Geometry check sheet. Reference: the model listing, model coordinates, mm. A direction names the side the tool comes from. Give positions to 0.01 mm unless a question says otherwise; leave off trailing zeros. Write each loop counter-clockwise with the first axis right and the second up, starting at its lowest first coordinate (ties: lowest second). Pieces come first, ordered by that corner, then holes.
(1) Mould release check, pull along Y, two halves, no side actions. Record for faces 1 (the cylindrical face through (7.777, -9.686, -2.718)), 2 (the flat face through (-5, 5, -4.5)), 3 (the cylindrical face through (-4.336, -19.524, -2.218)): +Y half, -Y half, draft (parallel to the pull), parting line (faces both ways), or undercut.
(2) Cross-section at A-A (y = 0). Record the boundary of the cut face in (x, z), and give its area (3 significant figures).
(3) Cross-section at D-D (y = 14). Record the boundary of the cut face in (x, z), and give its area (3 significant figures).
(4) Cross-section at C-C (x = 17.5). Record the boundary of the cut face in (y, z).
(5) Thickness scan on line 1 along Y through (x, z) = (0, -3.95); line 2 along Y through (x, z) = (-8, -3.45); line 3 along Z through (x, y) = (2.5, -8.5). Record the ranges inside material, lowest first.
(6) Tool access check on faces 4 (the cylindrical face through (10.16, -0.09, -1.48)), 5 (the flat face through (-4.7, 9.2, 0)). Record the directions out of +Z, -Z, +X, -X, +Y, -Y that give a thin tool (end or side, any length) a straight path to the whole face; none if there is none.
(7) Depth check by flat-ended pin: P1, Ø1.5, axis at y = -3.5, z = -3, coming from the +X side; P2, Ø22.5, axis at x = -3.5, y = -2, coming from the +Z side; P3, Ø3, axis at x = -8, y = -8.07, coming from the +Z side (3 decimals); P4, Ø1, axis at y = -3.5, z = -2.5, coming from the -X side. Enter the tip coordinate at first touch or a pass-through.
(8) Cross-section at B-B (x = -5). Record the boundary of the cut face in (y, z).
Autodesk Inventor part; units mm, degrees
ref_plane "YZ Plane" through (0, 0, 0) normal (1, 0, 0) x (0, 1, 0)
ref_plane "XZ Plane" through (0, 0, 0) normal (0, 1, 0) x (-1, 0, 0)
ref_plane "XY Plane" through (0, 0, 0) normal (0, 0, 1) x (1, 0, 0)
sketch "Sketch8" plane through (0, 0, 0) normal (0, 0, 1) x (1, 0, 0)
  circle A0 centre (0, 0) radius 15
  dimension "d33" = 30
extrude "Extrusion7" add sketch "Sketch8" against normal blind 8
sketch "Sketch10" plane through (0, 0, -8) normal (0, 0, -1) x (-1, 0, 0)
  line L0 (9, 10.07) -> (-29.1, 10.07)
  arc A0 (10, 9.07) -> (9, 10.07) centre (9, 9.07) ccw
  line L1 (10, 9.07) -> (10, -9.07)
  arc A1 (9, -10.07) -> (10, -9.07) centre (9, -9.07) ccw
  line L2 (-29.1, -10.07) -> (9, -10.07)
  line L3 (-29.1, 10.07) -> (-29.1, -10.07)
  line L4 (10.4, -9.07) -> (10.4, 9.07)
  arc A2 (10.4, 9.07) -> (9, 10.47) centre (9, 9.07) ccw
  line L5 (9, 10.47) -> (-29.5, 10.47)
  line L6 (-29.5, 10.47) -> (-29.5, -10.47)
  line L7 (-29.5, -10.47) -> (9, -10.47)
  arc A3 (9, -10.47) -> (10.4, -9.07) centre (9, -9.07) ccw
  dimension "d59" = 0.4
extrude "Extrusion8" cut sketch "Sketch10" against normal blind 2 contours A0 L1 A1 L2 L3 L0 | A3 L7 L6 L5 A2 L4
sketch "Sketch11" plane through (0, 0, -6) normal (0, 0, -1) x (-1, 0, 0)
  circle A0 centre (0, 0) radius 6.4
  circle A1 centre (0, 0) radius 6.5
  point P0 (0, 0)
  dimension "d58" = 13
extrude "Extrusion9" cut sketch "Sketch11" against normal through all contours A0 | A1
sketch "Sketch13" plane through (0, 0, 0) normal (0, 0, 1) x (1, 0, 0)
  circle A0 centre (0, 0) radius 9.96
  circle A1 centre (0, 0) radius 10.16
  point P0 (0, 0)
  dimension "d44" = 0.2
extrude "Extrusion11" cut sketch "Sketch13" against normal blind 3 contours A0 | A1
sketch "Sketch14" plane through (0, 0, 0) normal (0, 0, 1) x (1, 0, 0)
  circle A0 centre (6.9, 8) radius 0.7835
  circle A1 centre (6.9, -8) radius 0.7835
  circle A2 centre (-8, 8.07) radius 1
  circle A3 centre (-8, -8.07) radius 1
  point P0 (0, 0)
hole "Hole2" at (6.9, 8, 0) at (-8, 8.07, 0) at (-8, -8.07, 0) at (6.9, -8, 0) direction (0, 0, -1) diameter 2.1 end through all
sketch "Sketch15" plane through (0, 0, 0) normal (0, 0, 1) x (1, 0, 0)
  arc A0 (7.3255, 7.0401) -> (5.888, 8.2799) centre (6.9, 8) ccw
  arc A1 (5.888, -8.2799) -> (7.3255, -7.0401) centre (6.9, -8) ccw
  circle A2 centre (-8, 8.07) radius 1.05
  circle A3 centre (-8, -8.07) radius 1.05
  circle A4 centre (6.9, 8) radius 1.9
  circle A5 centre (6.9, -8) radius 1.9
  circle A6 centre (-8, -8.07) radius 1.9
  circle A7 centre (-8, 8.07) radius 1.9
  point P0 (0, 0)
  dimension "d54" = 3.8
extrude "Extrusion12" cut sketch "Sketch15" against normal blind 4.5 contours A2 | A3 | A4 | A5 | A6 | A7
fillet "Fillet2" radius 0.5 8 edges at (5.1562, 8.7544, -1.5) (7.9023, 6.3859, -1.5) (-6.1008, 8.1244, -1.5) (-8.071, 6.1713, -1.5) (-8.071, -6.1713, -1.5) (-6.1008, -8.1244, -1.5) (5.1562, -8.7544, -1.5) (7.9023, -6.3859, -1.5)
sketch "Sketch16" plane through (0, 0, -8) normal (0, 0, -1) x (-1, 0, 0)
  circle A0 centre (-6.9, -8) radius 1.05
  circle A1 centre (8, -8.07) radius 1.05
  circle A2 centre (8, 8.07) radius 1.05
  circle A3 centre (-6.9, 8) radius 1.05
  circle A4 centre (0, 0) radius 6.5
  arc A5 (-10.7415, 10.47) -> (-10.7415, -10.47) centre (0, 0) ccw
  line L0 (9, -10.47) -> (-10.7415, -10.47)
  arc A6 (9, -10.47) -> (10.4, -9.07) centre (9, -9.07) ccw
  line L1 (10.4, 9.07) -> (10.4, -9.07)
  arc A7 (10.4, 9.07) -> (9, 10.47) centre (9, 9.07) ccw
  line L2 (-10.7415, 10.47) -> (9, 10.47)
  line L3 (-10.7415, 10.47) -> (9, 10.47)
  arc A8 (10.4, 9.07) -> (9, 10.47) centre (9, 9.07) ccw
  line L4 (10.4, 9.07) -> (10.4, -9.07)
  arc A9 (9, -10.47) -> (10.4, -9.07) centre (9, -9.07) ccw
  line L5 (9, -10.47) -> (-10.7415, -10.47)
  arc A10 (-10.7415, -10.47) -> (-10.7415, 10.47) centre (0, 0) ccw
extrude "Extrusion14" cut sketch "Sketch16" against normal blind 3.5
sketch "Sketch19" plane through (0, 0, 0) normal (0, 0, 1) x (1, 0, 0)
  circle A0 centre (0, 0) radius 15
  circle A1 centre (0, 0) radius 20
  dimension "d67" = 30
  dimension "d68" = 40
extrude "Extrusion16" add sketch "Sketch19" against normal blind 4.5
properties part number "frame_motor_support" material "Aluminum 6061-AHC"
Reply:
1. face 1: undercut
1. face 2: draft
1. face 3: parting line
2. outline: (-20, -4.5) - (-6.5, -4.5) - (-6.5, -3) - (-10.16, -3) - (-10.16, 0) - (-20, 0) - close; (6.5, -4.5) - (20, -4.5) - (20, 0) - (10.16, 0) - (10.16, -3) - (6.5, -3) - close
2. area: 99.5 mm2
3. outline: (-14.28, -4.5) - (14.28, -4.5) - (14.28, 0) - (-14.28, 0) - close
3. area: 129 mm2
4. outline: (-9.68, -4.5) - (9.68, -4.5) - (9.68, 0) - (-9.68, 0) - close
5. line 1: y = -20 to -6.5, 6.5 to 20
5. line 2: y = -18.33 to -9.97, -6.17 to 6.17, 9.97 to 18.33
5. line 3: z = -4.5 to -3
6. face 4: +Z
6. face 5: +Z, +X, -X, +Y, -Y
7. P1: stops at x = 19.81
7. P2: stops at z = 0
7. P3: passes through
7. P4: stops at x = -19.77
8. outline: (-19.36, -4.5) - (-4.15, -4.5) - (-4.15, -3) - (-8.84, -3) - (-8.84, 0) - (-19.36, 0) - close; (4.15, -4.5) - (19.36, -4.5) - (19.36, 0) - (8.84, 0) - (8.84, -3) - (4.15, -3) - close
